```python
from build123d import *

# Parameters (mm, degrees)
SKETCH1_R           = 3
SKETCH1_R_2         = 19
BOSS_EXTRUDE1_DEPTH = 4
CUT_EXTRUDE1_DEPTH  = 5
SKETCH3_R           = 3.15
BOSS_EXTRUDE2_DEPTH = 4
FILLET1_R           = 5
SKETCH4_R           = 1.5
CUT_EXTRUDE2_DEPTH  = 5


with BuildPart() as part:
    # Sketch1 → Boss-Extrude1 (new body)
    with BuildSketch(Plane.XY):
        Polygon((0, 36.632796194), (-7.647271147, 32.990762303), (-9.405300929, 29.104152359), (-58.126981429, 27.62278105), (-76.5, 14.085859857), (-76.5, -14.085859857), (-58.126981429, -27.62278105), (-9.405300929, -29.104152359), (-7.647271147, -32.990762303), (0, -36.632796194), (7.647271147, -32.990762303), (9.405300929, -29.104152359), (58.126981429, -27.62278105), (76.5, -14.085859857), (76.5, 14.085859857), (58.126981429, 27.62278105), (9.405300929, 29.104152359), (7.647271147, 32.990762303), align=None)
        with Locations((0, 30)):
            Circle(SKETCH1_R, mode=Mode.SUBTRACT)
        with Locations((-50, 0)):
            Circle(SKETCH1_R_2, mode=Mode.SUBTRACT)
        with Locations((50, 0)):
            Circle(SKETCH1_R_2, mode=Mode.SUBTRACT)
        with Locations((0, -30)):
            Circle(SKETCH1_R, mode=Mode.SUBTRACT)
    extrude(amount=BOSS_EXTRUDE1_DEPTH)

    # Sketch2 → Cut-Extrude1 (cut, through all)
    with BuildSketch(Plane.XY.offset(4)):
        with BuildLine():
            Line((8.5, 20), (-8.5, 20))
            ThreePointArc((-8.5, 20), (-11.328427125, 18.828427125), (-12.5, 16))
            Line((-12.5, 16), (-12.5, -16))
            ThreePointArc((-12.5, -16), (-11.328427125, -18.828427125), (-8.5, -20))
            Line((-8.5, -20), (8.5, -20))
            ThreePointArc((8.5, -20), (11.328427125, -18.828427125), (12.5, -16))
            Line((12.5, -16), (12.5, 16))
            ThreePointArc((12.5, 16), (11.328427125, 18.828427125), (8.5, 20))
        make_face()
    extrude(amount=-CUT_EXTRUDE1_DEPTH, mode=Mode.SUBTRACT)

    # Sketch3 → Boss-Extrude2 (add)
    with BuildSketch(Plane.XY.offset(4)):
        Polygon((-58.126981429, 27.62278105), (-64.551915182, 31.10998542), (-77.245081729, 28.773819798), (-73.717039059, 16.136297176), align=None)
        with Locations((-70, 25)):
            Circle(SKETCH3_R, mode=Mode.SUBTRACT)
        Polygon((73.717039059, 16.136297176), (58.126981429, 27.62278105), (64.551915182, 31.10998542), (77.245081729, 28.773819798), align=None)
        with Locations((70, 25)):
            Circle(SKETCH3_R, mode=Mode.SUBTRACT)
        Polygon((58.126981429, -27.62278105), (64.551915182, -31.10998542), (77.245081729, -28.773819798), (73.717039059, -16.136297176), align=None)
        with Locations((70, -25)):
            Circle(SKETCH3_R, mode=Mode.SUBTRACT)
        Polygon((-73.717039059, -16.136297176), (-58.126981429, -27.62278105), (-64.551915182, -31.10998542), (-77.245081729, -28.773819798), align=None)
        with Locations((-70, -25)):
            Circle(SKETCH3_R, mode=Mode.SUBTRACT)
    extrude(amount=-BOSS_EXTRUDE2_DEPTH)

    # Fillet1
    fillet1_edges = [part.edges().sort_by_distance(p)[0] for p in [
        (77.245081729, 28.773819798, 2),
        (77.245081729, -28.773819798, 2),
        (-77.245081729, -28.773819798, 2),
        (-77.245081729, 28.773819798, 2),
    ]]
    fillet(fillet1_edges, radius=FILLET1_R)

    # Sketch4 → Cut-Extrude2 (cut, through all)
    with BuildSketch(Plane.XY.offset(4)):
        with Locations((-50, 23.75)):
            Circle(SKETCH4_R)
        with Locations((-70.56810334, 11.875)):
            Circle(SKETCH4_R)
        with Locations((-70.56810334, -11.875)):
            Circle(SKETCH4_R)
        with Locations((-50, -23.75)):
            Circle(SKETCH4_R)
        with Locations((-29.43189666, -11.875)):
            Circle(SKETCH4_R)
        with Locations((-29.43189666, 11.875)):
            Circle(SKETCH4_R)
        with Locations((29.43189666, 11.875)):
            Circle(SKETCH4_R)
        with Locations((29.43189666, -11.875)):
            Circle(SKETCH4_R)
        with Locations((50, -23.75)):
            Circle(SKETCH4_R)
        with Locations((70.56810334, -11.875)):
            Circle(SKETCH4_R)
        with Locations((70.56810334, 11.875)):
            Circle(SKETCH4_R)
        with Locations((50, 23.75)):
            Circle(SKETCH4_R)
    extrude(amount=-CUT_EXTRUDE2_DEPTH, mode=Mode.SUBTRACT)


solid = part.part
```
Check sheet for the modelled part. Datum: model origin and axes. Units: mm. A direction names the side the tool comes from. Give positions to 0.01 mm unless a question says otherwise; leave off trailing zeros. Write each loop counter-clockwise with the first axis right and the second up, starting at its lowest first coordinate (ties: lowest second). Pieces come first, ordered by that corner, then holes.
Item 1: Scan lines: L1, parallel to X at y = -16.5, z = 1.15; L2, parallel to Y at x = -50, z = 1.95; L3, parallel to X at y = -10, z = 0.8. Record each from-to range of solid material in increasing order.
Item 2: Access from +Z, -Z, +X, -X, +Y, -Y to the whole of each face (thin tool, end or side, straight path). Record for faces 1 (the face through (-68.156, -30.447, 2.028)), 2 (the face through (-11.297, 18.859, 2.028)).
Item 3: Cross-section at B-B (z = 3.1). Count the separate pieces of the cut face and the enclosed holes in it, and give its area (3 significant figures).
Item 4: Gauge pin test, flat ends, axial feed: pin 1 (2 mm diameter, centred on x = -39.5, z = 3, fed in from -Y); pin 2 (1 mm diameter, centred on y = -29, z = 1.5, fed in from +X); pin 3 (1 mm diameter, centred on y = -24.5, z = 1, fed in from -X). Record the tip position at first contact, or that the pin passes through.
Item 5: Cross-section at A-A (x = 41.5). Enter the section's corners in (y, z).
Item 6: Draft check along Y on faces 3 (the face through (48.89, -22.74, 2.03)), 4 (the face through (-8.54, -31.02, 1.97)), 5 (the face through (69.07, -11.81, 2.03)), 6 (the face through (-18, 1, 4)). Enter one of: released by +Y, released by -Y, zero draft, split by the parting line, or undercut.
Report:
1. L1: x = -73.82 to -59.42, -40.58 to -12.47, 12.47 to 40.58, 59.42 to 73.82
1. L2: y = -27.87 to -25.25, -22.25 to -19, 19 to 22.25, 25.25 to 27.87
1. L3: x = -76.5 to -66.16, -33.84 to -12.5, 12.5 to 33.84, 66.16 to 76.5
2. face 1: +Z, -Z, -X, -Y
2. face 2: +Z, -Z
3. separate pieces: 1
3. enclosed holes: 21
3. area: 5,390 mm2
4. pin 1: stops at y = -28.22
4. pin 2: stops at x = 74.37
4. pin 3: stops at x = -75.96
5. outline: (-28.13, 0) - (-16.99, 0) - (-16.99, 4) - (-28.13, 4) - close; (16.99, 0) - (28.13, 0) - (28.13, 4) - (16.99, 4) - close
6. face 3: undercut
6. face 4: released by -Y
6. face 5: undercut
6. face 6: zero draft
